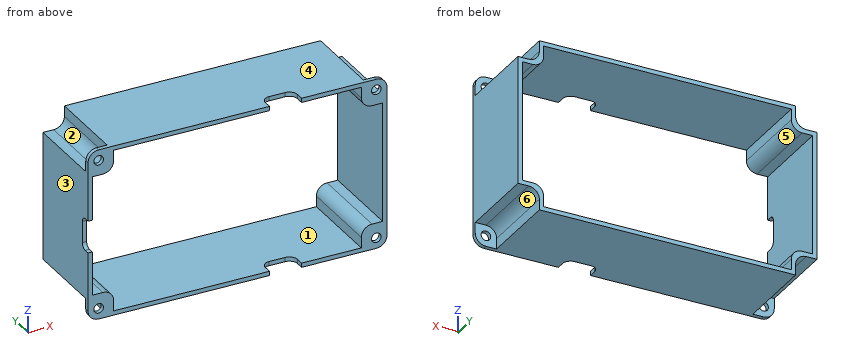
```python
from build123d import *

# Parameters (mm, degrees)
SKETCH1_W           = 116
SKETCH1_H           = 2
SKETCH1_W_2         = 2
SKETCH1_H_2         = 56
BOSS_EXTRUDE6_DEPTH = 40
SKETCH1_7_W         = 10
SKETCH1_7_H         = 10
SKETCH1_7_R         = 2.25
BOSS_EXTRUDE7_DEPTH = 2
FILLET1_R           = 5
CUT_EXTRUDE1_DEPTH  = 114.578166916
CUT_EXTRUDE2_REACH  = 152.997


with BuildPart() as part:
    # Sketch1 → Boss-Extrude6 (new body)
    with BuildSketch(Plane(origin=(0, 0, 0), x_dir=(1, 0, 0), z_dir=(0, 1, 0))):
        with Locations((0, -39)):
            Rectangle(SKETCH1_W, SKETCH1_H)
        Polygon((70, -30), (70, -28), (68, -28), (58, -28), (58, -38), (58, -40), (60, -40), (60, -30), align=None)
        with Locations((69, 0)):
            Rectangle(SKETCH1_W_2, SKETCH1_H_2)
        Polygon((70, 28), (70, 30), (60, 30), (60, 40), (58, 40), (58, 38), (58, 28), (68, 28), align=None)
        with Locations((0, 39)):
            Rectangle(SKETCH1_W, SKETCH1_H)
        Polygon((-58, 38), (-58, 40), (-60, 40), (-60, 30), (-70, 30), (-70, 28), (-68, 28), (-58, 28), align=None)
        with Locations((-69, 0)):
            Rectangle(SKETCH1_W_2, SKETCH1_H_2)
        Polygon((-58, -40), (-58, -38), (-58, -28), (-68, -28), (-70, -28), (-70, -30), (-60, -30), (-60, -40), align=None)
    extrude(amount=BOSS_EXTRUDE6_DEPTH)

    # Sketch1_7 → Boss-Extrude7 (add)
    # profile 1 of 4: a face of its own
    with BuildSketch(Plane(origin=(0, 0, 0), x_dir=(1, 0, 0), z_dir=(0, 1, 0))):
        with Locations((-65, -35)):
            Rectangle(SKETCH1_7_W, SKETCH1_7_H)
        with Locations(Location((-65, -35, 0), (0, 0, 270))):
            Circle(SKETCH1_7_R, mode=Mode.SUBTRACT)
    # profile 2 of 4: a face of its own
    with BuildSketch(Plane(origin=(0, 0, 0), x_dir=(1, 0, 0), z_dir=(0, 1, 0))):
        with Locations((65, -35)):
            Rectangle(SKETCH1_7_W, SKETCH1_7_H)
        with Locations(Location((65, -35, 0), (0, 0, 270))):
            Circle(SKETCH1_7_R, mode=Mode.SUBTRACT)
    # profile 3 of 4: a face of its own
    with BuildSketch(Plane(origin=(0, 0, 0), x_dir=(1, 0, 0), z_dir=(0, 1, 0))):
        with Locations((65, 35)):
            Rectangle(SKETCH1_7_W, SKETCH1_7_H)
        with Locations(Location((65, 35, 0), (0, 0, 270))):
            Circle(SKETCH1_7_R, mode=Mode.SUBTRACT)
    # profile 4 of 4: a face of its own
    with BuildSketch(Plane(origin=(0, 0, 0), x_dir=(1, 0, 0), z_dir=(0, 1, 0))):
        with Locations((-65, 35)):
            Rectangle(SKETCH1_7_W, SKETCH1_7_H)
        with Locations(Location((-65, 35, 0), (0, 0, 270))):
            Circle(SKETCH1_7_R, mode=Mode.SUBTRACT)
    extrude(amount=BOSS_EXTRUDE7_DEPTH)

    # Fillet1
    fillet1_edges = [part.edges().sort_by_distance(p)[0] for p in [
        (70, 1, -40),
        (-70, 1, -40),
        (60, 21, -30),
        (60, 21, 30),
        (-60, 21, 30),
        (-60, 21, -30),
        (-58, 20, -28),
        (-58, 20, 28),
        (58, 20, 28),
        (58, 20, -28),
        (-70, 1, 40),
        (70, 1, 40),
    ]]
    fillet(fillet1_edges, radius=FILLET1_R)

    # Sketch2 → Cut-Extrude1 (cut, through all)
    with BuildSketch(Plane(origin=(0, 0, -40), x_dir=(-1, 0, 0), z_dir=(0, 0, -1))):
        with BuildLine():
            Line((-30, 0), (-15, 0))
            Line((-15, 0), (-15, 3.75))
            ThreePointArc((-15, 3.75), (-16.098349571, 6.401650429), (-18.75, 7.5))
            Line((-18.75, 7.5), (-26.25, 7.5))
            ThreePointArc((-26.25, 7.5), (-28.901650429, 6.401650429), (-30, 3.75))
            Line((-30, 3.75), (-30, 0))
        make_face()
    extrude(amount=-CUT_EXTRUDE1_DEPTH, mode=Mode.SUBTRACT)

    # Sketch3 → Cut-Extrude2 (cut, up to next)
    with BuildSketch(Plane.ZY.offset(70), mode=Mode.PRIVATE) as cut_extrude2_sk1:
        with BuildLine():
            Line((-7.5, 0), (7.5, 0))
            Line((7.5, 0), (7.5, 2.5))
            ThreePointArc((7.5, 2.5), (6.767766953, 4.267766953), (5, 5))
            Line((5, 5), (-5, 5))
            ThreePointArc((-5, 5), (-6.767766953, 4.267766953), (-7.5, 2.5))
            Line((-7.5, 2.5), (-7.5, 0))
        make_face()
    cut_extrude2_tool1 = extrude(cut_extrude2_sk1.sketch, amount=-CUT_EXTRUDE2_REACH, mode=Mode.PRIVATE) & part.part
    add(cut_extrude2_tool1.solids().sort_by_distance((-70, 2.42798, 0))[0], mode=Mode.SUBTRACT)


solid = part.part
```
The listing builds one solid part. Answer for the finished solid, in the listing's coordinates (mm). Face numbers are marked on the shaded views. A direction names the side the tool comes from. Coordinates: 2 decimals unless noted, no trailing zeros. Order: outer loops, then holes, each group sorted by start corner. A loop starts at its lowest first (then second) coordinate and runs counter-clockwise, first axis right, second up. Notation, with made-up numbers: M 11,-8.5 L 60,-8.5 A17 cw 60,24.5 Z; hole C 87.25,70 d5. An arc over 180 degrees is marked long. Answer as a JSON object with one key per item and string values. Group by question number.
1. Section B-B on z = 26.5 is taken. Write down the section's boundary in (x, y).
2. Section A-A on x = -49 is taken. Write down the section's boundary in (y, z), then the cut area to 3 significant figures.
3. Determine the mould class of the marked faces 1, 2 and 3 for opening direction Z: released by +Z, released by -Z, zero draft, split by the parting line, or undercut.
4. Straight lines are drawn through the part: line 1 (X direction, y = 1, z = 35); line 2 (Z direction, x = 5, y = 32.5); line 3 (X direction, y = 15.5, z = -19). For each, find the intervals that lie inside material, in ascending order.
5. Flat-ended cylindrical pins translate along their axes: P1, Ø0.6, axis at y = 2, z = -39, coming from the +X side; P2, Ø2.5, axis at x = -67, y = 24, coming from the +Z side; P3, Ø2, axis at x = -68.5, y = 1, coming from the -Z side. Find the tip coordinate at first contact, or state that the pin passes through.
6. A tool of negligible diameter and unlimited length cuts with its end or side. For the marked faces 4, 5 and 6, from which of +Z, -Z, +X, -X, +Y, -Y can it reach the whole face along a straight path? Write none if from no direction.
Values follow:
{
 "1": {"outline": "M -70,0 L -68,0 L -68,40 L -70,40 Z; M 68,0 L 70,0 L 70,40 L 68,40 Z"},
 "2": {"outline": "M 0,-40 L 40,-40 L 40,-38 L 0,-38 Z; M 0,38 L 40,38 L 40,40 L 0,40 Z", "area": "160 mm2"},
 "3": {"face 1": "undercut", "face 2": "released by +Z", "face 3": "zero draft"},
 "4": {"line 1": "-70 to -67.25, -62.75 to -58, 58 to 62.75, 67.25 to 70", "line 2": "-40 to -38, 38 to 40", "line 3": "-70 to -68, 68 to 70"},
 "5": {"P1": "x = 68.36", "P2": "z = 30", "P3": "z = -39.33"},
 "6": {"face 4": "+Z, +X, -X, +Y, -Y", "face 5": "+Y, -Y", "face 6": "-Z, +X, +Y"}
}
